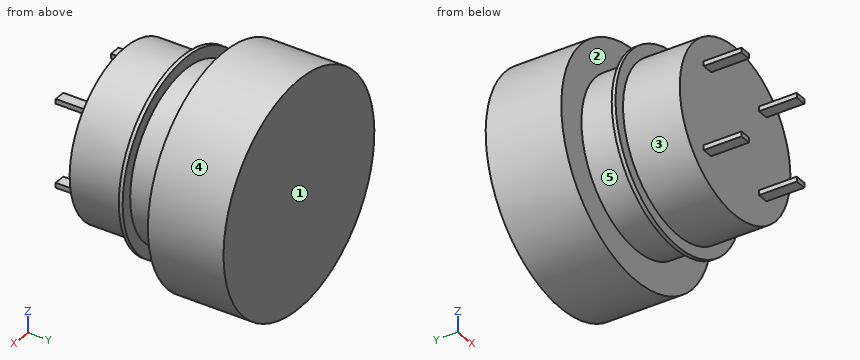
```python
from build123d import *

# Parameters (mm, degrees)
ESQUISSE1_R        = 22
BOSS_EXTRU_1_DEPTH = 15
ESQUISSE2_R        = 25
BOSS_EXTRU_2_DEPTH = 1
ESQUISSE3_R        = 22
BOSS_EXTRU_3_DEPTH = 10
ESQUISSE4_R        = 30
BOSS_EXTRU_4_DEPTH = 20
ESQUISSE5_W        = 3
ESQUISSE5_H        = 1.260124144
ESQUISSE5_H_2      = 1.295969654
BOSS_EXTRU_5_DEPTH = 10


with BuildPart() as part:
    # Esquisse1 → Boss.-Extru.1 (new body)
    with BuildSketch(Plane(origin=(0, 0, 0), x_dir=(1, 0, 0), z_dir=(0, 1, 0))):
        with Locations(Location((0, 0, 0), (0, 0, 270))):
            Circle(ESQUISSE1_R)
    extrude(amount=BOSS_EXTRU_1_DEPTH)

    # Esquisse2 → Boss.-Extru.2 (add)
    with BuildSketch(Plane(origin=(0, 15, 0), x_dir=(1, 0, 0), z_dir=(0, 1, 0))):
        with Locations(Location((0, 0, 0), (0, 0, 270))):
            Circle(ESQUISSE2_R)
    extrude(amount=BOSS_EXTRU_2_DEPTH)

    # Esquisse3 → Boss.-Extru.3 (add)
    with BuildSketch(Plane(origin=(0, 16, 0), x_dir=(1, 0, 0), z_dir=(0, 1, 0))):
        with Locations(Location((0, 0, 0), (0, 0, 270))):
            Circle(ESQUISSE3_R)
    extrude(amount=BOSS_EXTRU_3_DEPTH)

    # Esquisse4 → Boss.-Extru.4 (add)
    with BuildSketch(Plane(origin=(0, 26, 0), x_dir=(1, 0, 0), z_dir=(0, 1, 0))):
        with Locations(Location((0, 0, 0), (0, 0, 270))):
            Circle(ESQUISSE4_R)
    extrude(amount=BOSS_EXTRU_4_DEPTH)

    # Esquisse5 → Boss.-Extru.5 (add)
    with BuildSketch(Plane.XZ):
        with Locations((-11, 11)):
            Rectangle(ESQUISSE5_W, ESQUISSE5_H)
        with Locations((-11, -11)):
            Rectangle(ESQUISSE5_W, ESQUISSE5_H_2)
        with Locations((11, -11)):
            Rectangle(ESQUISSE5_W, ESQUISSE5_H_2)
        with Locations((11, 11)):
            Rectangle(ESQUISSE5_W, ESQUISSE5_H)
    extrude(amount=BOSS_EXTRU_5_DEPTH)


solid = part.part
```
Work out the finished part from the listing and answer in its coordinate system (mm). Face numbers are marked on the shaded views. A direction names the side the tool comes from. Give positions to 0.01 mm unless a question says otherwise; leave off trailing zeros. Order: outer loops, then holes, each group sorted by start corner. A loop starts at its lowest first (then second) coordinate and runs counter-clockwise, first axis right, second up. Notation, with made-up numbers: (79.5, 76.5) -> (127.5, 76.5) arc R29 cw to (127.5, 97.5) -> close; hole circle Ø11 at (-24, -18). An arc over 180 degrees is marked (long way). Answer as CSV lines item,"result". Start each with the question number.
(1) Section B-B, the plane x = 0 is taken. Write down the section's boundary in (y, z).
(2) Which of the six approach directions +Z, -Z, +X, -X, +Y, -Y give full straight-line access (tool end or side, diameter ignored) to the marked faces 4 and 5?
(3) Consider line 1 along Y through (x, z) = (23, 7); line 2 along Y through (x, z) = (25, -6.5); line 3 along Y through (x, z) = (7, 4.5). Determine where each line is inside the solid, lowest interval first.
(4) Section A-A, the plane y = -6 is taken. Write down the section's boundary in (x, z).
(5) Section D-D, the plane y = 20 is taken. Write down the section's boundary in (x, z).
(6) Section C-C, the plane z = 0 is taken. Write down the section's boundary in (x, y).
(7) For a pull along Y with two mould halves and no side action, classify the marked faces 1, 2 and 3 as released by +Y, released by -Y, zero draft, split by the parting line, or undercut.
(8) Each of these flat-tipped pins is pushed along its axis until it touches: pin 1 Ø2.5 at (x, y) = (-10.5, -5) entering from +Z; pin 2 Ø6 at (y, z) = (10.5, -5) entering from -X; pin 3 Ø12 at (x, y) = (-10, 35.5) entering from +Z; pin 4 Ø18 at (x, z) = (3, 5) entering from -Y. Where does it stop, or does it pass through?
Entries:
1,outline,"(0, -22) -> (15, -22) -> (15, -25) -> (16, -25) -> (16, -22) -> (26, -22) -> (26, -30) -> (46, -30) -> (46, 30) -> (26, 30) -> (26, 22) -> (16, 22) -> (16, 25) -> (15, 25) -> (15, 22) -> (0, 22) -> close"
2,face 4,"+Y, -Y"
2,face 5,"none"
3,line 1,"15 to 16, 26 to 46"
3,line 2,"26 to 46"
3,line 3,"0 to 46"
4,outline,"(-12.5, -11.65) -> (-9.5, -11.65) -> (-9.5, -10.35) -> (-12.5, -10.35) -> close; (-12.5, 10.37) -> (-9.5, 10.37) -> (-9.5, 11.63) -> (-12.5, 11.63) -> close; (9.5, -11.65) -> (12.5, -11.65) -> (12.5, -10.35) -> (9.5, -10.35) -> close; (9.5, 10.37) -> (12.5, 10.37) -> (12.5, 11.63) -> (9.5, 11.63) -> close"
5,outline,"circle Ø44 at (0, 0)"
6,outline,"(-30, 26) -> (-22, 26) -> (-22, 16) -> (-25, 16) -> (-25, 15) -> (-22, 15) -> (-22, 0) -> (22, 0) -> (22, 15) -> (25, 15) -> (25, 16) -> (22, 16) -> (22, 26) -> (30, 26) -> (30, 46) -> (-30, 46) -> close"
7,face 1,"released by +Y"
7,face 2,"undercut"
7,face 3,"zero draft"
8,pin 1,"z = 11.63"
8,pin 2,"x = -21.91"
8,pin 3,"z = 29.73"
8,pin 4,"y = -10"
